```python
from build123d import *

# Parameters (mm, degrees)
SKETCH1_R           = 6.35
BOSS_EXTRUDE1_DEPTH = 19.05


with BuildPart() as part:
    # Sketch1 → Boss-Extrude1 (new body)
    with BuildSketch(Plane.XY):
        Polygon((-1.304733728, 61.99852071), (-1.304733728, -1.50147929), (11.395266272, -1.50147929), (11.395266272, 11.19852071), (74.895266272, 11.19852071), (74.895266272, -1.50147929), (87.595266272, -1.50147929), (87.595266272, 36.59852071), (49.495266272, 61.99852071), align=None)
        with Locations((24.095266272, 36.59852071)):
            Circle(SKETCH1_R, mode=Mode.SUBTRACT)
        with Locations((55.845266272, 36.59852071)):
            Circle(SKETCH1_R, mode=Mode.SUBTRACT)
    extrude(amount=BOSS_EXTRUDE1_DEPTH)


solid = part.part
```
Can you work these out from the model? Positions are in its coordinate system, mm. A direction names the side the tool comes from. Coordinates: 2 decimals unless noted, no trailing zeros. Loops run counter-clockwise (first coordinate to the right, second up) from the corner with the lowest first, then second, coordinate; pieces in that order, holes last.
Item 1: Suppose I cut it at D-D (y = 34). Please give me the cut outline in (x, z).
Answers below:
outline: (-1.3, 0) - (18.3, 0) - (18.3, 19.05) - (-1.3, 19.05) - close; (29.89, 0) - (50.05, 0) - (50.05, 19.05) - (29.89, 19.05) - close; (61.64, 0) - (87.6, 0) - (87.6, 19.05) - (61.64, 19.05) - close
Item 2: Which directions (+Z, -Z, +X, -X, +Y, -Y) give clear straight access to the entire face, cutting with the end or side of a thin tool? Please do faces 1 (the face through (11.395, 5, 9)), 2 (the face through (87.595, 17, 9)).
Answers below:
face 1: +Z, -Z, -Y
face 2: +Z, -Z, +X, +Y, -Y
Item 3: I'm going to push a flat-ended pin straight in: pin 1 (1 mm diameter, centred on x = 60, z = 7, fed in from +Y). Where does the tip first touch, or does it pass through?
Answers below:
pin 1: stops at y = 55.33
Item 4: Suppose I cut it at A-A (z = 1.5). Please give me the cut outline in (x, y).
Answers below:
outline: (-1.3, -1.5) - (11.4, -1.5) - (11.4, 11.2) - (74.9, 11.2) - (74.9, -1.5) - (87.6, -1.5) - (87.6, 36.6) - (49.5, 62) - (-1.3, 62) - close; hole circle Ø12.7 at (24.1, 36.6); hole circle Ø12.7 at (55.85, 36.6)
Item 5: Suppose I cut it at B-B (y = 10). Please give me the cut outline in (x, z).
Answers below:
outline: (-1.3, 0) - (11.4, 0) - (11.4, 19.05) - (-1.3, 19.05) - close; (74.9, 0) - (87.6, 0) - (87.6, 19.05) - (74.9, 19.05) - close
Item 6: Please list where these lines run through material, in increasing order: L1, parallel to X at y = 6, z = 11.75; L2, parallel to X at y = 41.5, z = 7; L3, parallel to X at y = 31.5, z = 10.75.
Answers below:
L1: x = -1.3 to 11.4, 74.9 to 87.6
L2: x = -1.3 to 20.06, 28.13 to 51.81, 59.88 to 80.24
L3: x = -1.3 to 20.31, 27.88 to 52.06, 59.63 to 87.6
Item 7: If we mould it in two halves opening along X, with no side actions, what happens to faces 3 (the face through (43, 31, 19.05)), 4 (the face through (68.81, 49.12, 9.39)), 5 (the face through (74.895, 5, 9))? For each: released by +X, released by -X, zero draft, split by the parting line, or undercut.
Answers below:
face 3: zero draft
face 4: released by +X
face 5: undercut
Item 8: Suppose I cut it at C-C (x = 51.5). Please give me the cut outline in (y, z).
Answers below:
outline: (11.2, 0) - (31.97, 0) - (31.97, 19.05) - (11.2, 19.05) - close; (41.23, 0) - (60.66, 0) - (60.66, 19.05) - (41.23, 19.05) - close
